Study the drawing (mm; zero at the part's minimum x, y, z) and answer. Coordinates: 2 decimals unless noted, no trailing zeros. Write each loop counter-clockwise with the first axis right and the second up, starting at its lowest first coordinate (ties: lowest second). Pieces come first, ordered by that corner, then holes. Notation, with made-up numbers: (-22.5, 43.25) -> (11.5, 43.25) arc R22 cw to (11.5, 52.25) -> close; hole circle Ø6 at (84, 12). An arc over 180 degrees is marked (long way). Answer in a Markdown table with one row per item. Add a question column.
Item 1: Straight lines are drawn through the part: line 1 (X direction, y = 47, z = 8); line 2 (X direction, y = 58.5, z = 18.5); line 3 (Y direction, x = 75, z = 11.25). For each, find the intervals that lie inside material, in ascending order. Write a range as from..to.
Item 2: Section D-D on y = 15.5 is taken. Write down the section's boundary in (x, z).
Item 3: Section C-C on z = 17 is taken. Write down the section's boundary in (x, y), then the cut area to 3 significant figures.
Item 4: Section A-A on x = 25 is taken. Write down the section's boundary in (y, z).
Item 5: Section B-B on y = 50 is taken. Write down the section's boundary in (x, z), then the cut area to 3 significant figures.
Item 6: For a pull along Y with two mould halves and no side action, classify the marked faces 1, 2 and 3 as +Y half, -Y half, draft (parallel to the pull), parting line (faces both ways), or undercut.
Item 7: Given pin 1 Ø12 at (x, y) = (146.5, 37.5) entering from +Z; pin 2 Ø1.5 at (y, z) = (56.5, 23) entering from +X, each flat-ended and moving along its own axis, determine where each tip first touches the part or whether it passes through.
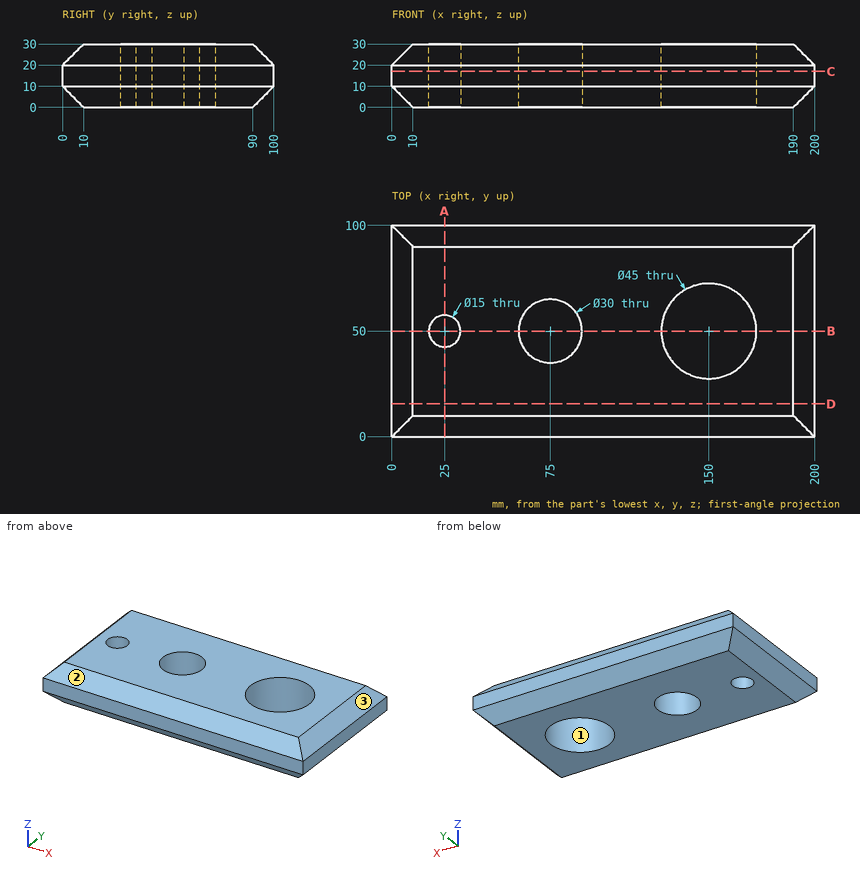
Results below:
| question | item | result |
|---|---|---|
| 1 | line 1 | x = 2..18.13, 31.87..60.3, 89.7..127.7, 172.3..198 |
| 1 | line 2 | x = 0..62.64, 87.36..129.17, 170.83..200 |
| 1 | line 3 | y = 0..35, 65..100 |
| 2 | outline | (0, 10) -> (10, 0) -> (190, 0) -> (200, 10) -> (200, 20) -> (190, 30) -> (10, 30) -> (0, 20) -> close |
| 3 | outline | (0, 0) -> (200, 0) -> (200, 100) -> (0, 100) -> close; hole circle Ø15 at (25, 50); hole circle Ø30 at (75, 50); hole circle Ø45 at (150, 50) |
| 3 | area | 17,500 mm2 |
| 4 | outline | (0, 10) -> (10, 0) -> (42.5, 0) -> (42.5, 30) -> (10, 30) -> (0, 20) -> close; (57.5, 0) -> (90, 0) -> (100, 10) -> (100, 20) -> (90, 30) -> (57.5, 30) -> close |
| 5 | outline | (0, 10) -> (10, 0) -> (17.5, 0) -> (17.5, 30) -> (10, 30) -> (0, 20) -> close; (32.5, 0) -> (60, 0) -> (60, 30) -> (32.5, 30) -> close; (90, 0) -> (127.5, 0) -> (127.5, 30) -> (90, 30) -> close; (172.5, 0) -> (190, 0) -> (200, 10) -> (200, 20) -> (190, 30) -> (172.5, 30) -> close |
| 5 | area | 3,100 mm2 |
| 6 | face 1 | undercut |
| 6 | face 2 | -Y half |
| 6 | face 3 | draft |
| 7 | pin 1 | passes through |
| 7 | pin 2 | stops at x = 197.75 |
